Source: three-view drawing plus pictorial views. Frame: mm from the lowest corner of the part. Give positions to 0.01 mm unless a question says otherwise; leave off trailing zeros. Order: outer loops, then holes, each group sorted by start corner. A loop starts at its lowest first (then second) coordinate and runs counter-clockwise, first axis right, second up. Notation, with made-up numbers: (-31.75, -17) -> (5.25, -17) arc R18 ccw to (5.25, -10) -> close; hole circle Ø11 at (-28, 54.25). An arc over 180 degrees is marked (long way). Use a Markdown table: item, result. Add a question column.
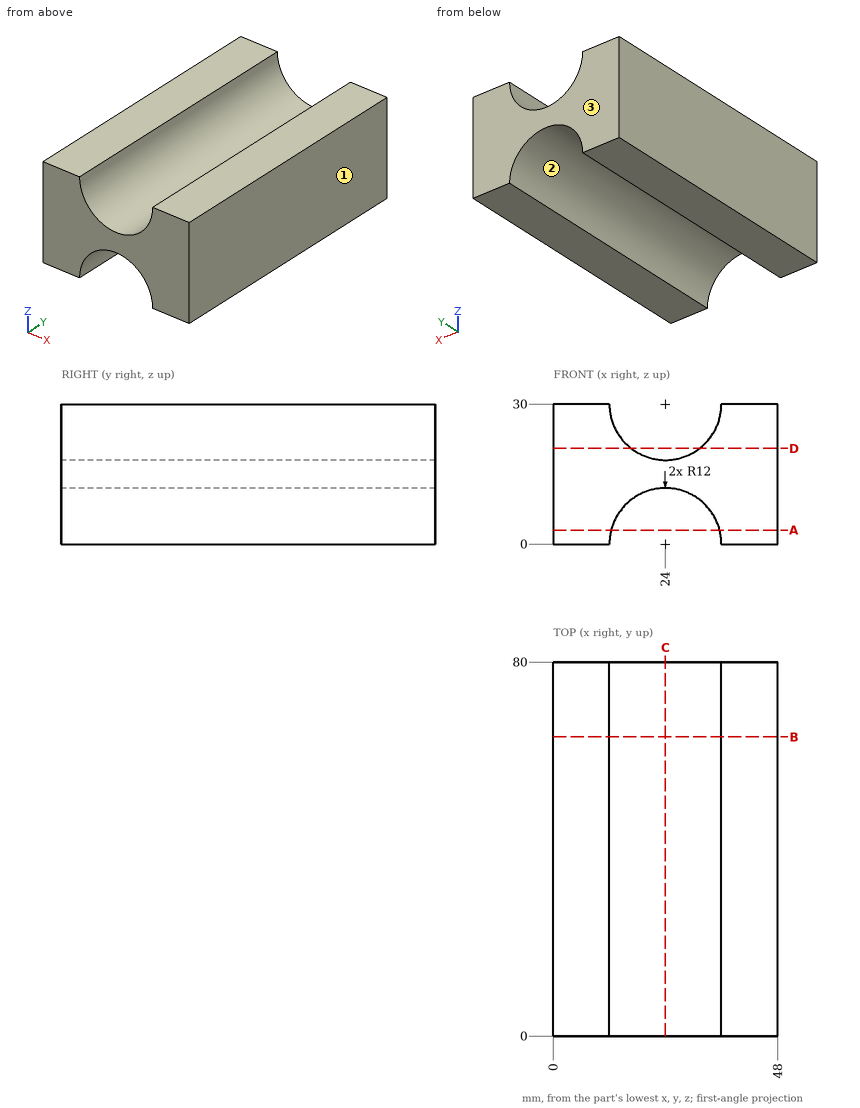
Q1. Ray query, line 1 (X direction, y = 8.5, z = 8.5); line 2 (X direction, y = 35.5, z = 19.5); line 3 (Z direction, x = 24, y = 71). Return the intervals inside material, ascending.
Q2. Section query C-C (x = 24). Return loops of the section in (y, z).
Q3. Section query D-D (z = 20.5). Return loops of the section in (x, y).
Q4. Section query A-A (z = 3). Return loops of the section in (x, y).
Q5. Draft query along X for the marked faces 1, 2 and 3. Return one class per face: +X half, -X half, draft (parallel to the pull), parting line (faces both ways), or undercut.
Q6. First-contact query: pin 1 (12 mm diameter, centred on y = 58.5, z = 24, fed in from -X); pin 2 (6 mm diameter, centred on x = 31.5, y = 32.5, fed in from +Z). Flat tips, straight axial feed; report the tip coordinate or a pass-through.
Q7. Section query B-B (y = 64). Return loops of the section in (x, z), plus the area to 3 significant figures.
Solution:
| question | item | result |
|---|---|---|
| 1 | line 1 | x = 0 to 15.53, 32.47 to 48 |
| 1 | line 2 | x = 0 to 18.19, 29.81 to 48 |
| 1 | line 3 | z = 12 to 18 |
| 2 | outline | (0, 12) -> (80, 12) -> (80, 18) -> (0, 18) -> close |
| 3 | outline | (0, 0) -> (16.67, 0) -> (16.67, 80) -> (0, 80) -> close; (31.33, 0) -> (48, 0) -> (48, 80) -> (31.33, 80) -> close |
| 4 | outline | (0, 0) -> (12.38, 0) -> (12.38, 80) -> (0, 80) -> close; (35.62, 0) -> (48, 0) -> (48, 80) -> (35.62, 80) -> close |
| 5 | face 1 | +X half |
| 5 | face 2 | undercut |
| 5 | face 3 | draft |
| 6 | pin 1 | stops at x = 0 |
| 6 | pin 2 | stops at z = 24.19 |
| 7 | outline | (0, 0) -> (12, 0) arc R12 cw to (36, 0) -> (48, 0) -> (48, 30) -> (36, 30) arc R12 cw to (12, 30) -> (0, 30) -> close |
| 7 | area | 988 mm² |
